The listing builds one solid part. Answer for the finished solid, in the listing's coordinates (mm). A direction names the side the tool comes from. Coordinates: 2 decimals unless noted, no trailing zeros. Loops run counter-clockwise (first coordinate to the right, second up) from the corner with the lowest first, then second, coordinate; pieces in that order, holes last. Notation, with made-up numbers: (-40, 38.5) -> (11, 38.5) arc R10 cw to (11, 52.5) -> close; hole circle Ø10 at (-39.75, 51.25). An arc over 180 degrees is marked (long way). Answer in a Markdown table with one row per item.
```python
from build123d import *

# Parameters (mm, degrees)
BOSS_EXTRUDE1_DEPTH      = 1.2
SKETCH2_R                = 1.5
CUT_EXTRUDE1_DEPTH       = 19.437461864
BOSS_EXTRUDE2_DEPTH      = 2.5
BOSS_EXTRUDE3_DEPTH      = 5.5
BOSS_EXTRUDE3_DEPTH_BACK = 4.7
SKETCH6_W                = 0.5
SKETCH6_H                = 0.5
SKETCH7_W                = 16
SKETCH7_H                = 26.8
BOSS_EXTRUDE4_DEPTH      = 1.8
SKETCH8_W                = 1.5
SKETCH8_H                = 0.75
SKETCH8_W_2              = 0.75
SKETCH8_H_2              = 1.5
BOSS_EXTRUDE5_DEPTH      = 0.8
SKETCH10_W               = 0.1
SKETCH10_H               = 8
BOSS_EXTRUDE6_DEPTH      = 0.1
SKETCH12_W               = 1
SKETCH12_H               = 22.2
BOSS_EXTRUDE7_DEPTH      = 0.06


with BuildPart() as part:
    # Sketch1 → Boss-Extrude1 (new body)
    with BuildSketch(Plane.XY):
        Polygon((10, -8.5), (10, 8.5), (12.5, 8.5), (12.5, 13.5), (-12.5, 13.5), (-12.5, -13.5), (12.5, -13.5), (12.5, -8.5), align=None)
    extrude(amount=BOSS_EXTRUDE1_DEPTH)

    # Sketch2 → Cut-Extrude1 (cut, through all)
    with BuildSketch(Plane.XY.offset(1.2)):
        with Locations((10.5, 11.5)):
            Circle(SKETCH2_R)
        with Locations(Location((10.5, -11.5, 0), (0, 0, 180))):
            Circle(SKETCH2_R)
        with Locations(Location((-10.5, 11.5, 0), (0, 0, 180))):
            Circle(SKETCH2_R)
        with Locations((-10.5, -11.5)):
            Circle(SKETCH2_R)
    extrude(amount=-CUT_EXTRUDE1_DEPTH, mode=Mode.SUBTRACT)

    # Sketch5 → Boss-Extrude2 (add)
    with BuildSketch(Plane(origin=(0, 0, 0), x_dir=(-1, 0, 0), z_dir=(0, 0, -1))):
        with BuildLine():
            Line((12.05, 6), (9.95, 6))
            ThreePointArc((9.95, 6), (9.808578644, 5.941421356), (9.75, 5.8))
            Line((9.75, 5.8), (9.75, 3.7))
            ThreePointArc((9.75, 3.7), (9.808578644, 3.558578644), (9.95, 3.5))
            ThreePointArc((9.95, 3.5), (9.808578644, 3.441421356), (9.75, 3.3))
            Line((9.75, 3.3), (9.75, 1.2))
            ThreePointArc((9.75, 1.2), (9.808578644, 1.058578644), (9.95, 1))
            ThreePointArc((9.95, 1), (9.808578644, 0.941421356), (9.75, 0.8))
            Line((9.75, 0.8), (9.75, -1.3))
            ThreePointArc((9.75, -1.3), (9.808578644, -1.441421356), (9.95, -1.5))
            ThreePointArc((9.95, -1.5), (9.808578644, -1.558578644), (9.75, -1.7))
            Line((9.75, -1.7), (9.75, -3.8))
            ThreePointArc((9.75, -3.8), (9.808578644, -3.941421356), (9.95, -4))
            Line((9.95, -4), (12.05, -4))
            ThreePointArc((12.05, -4), (12.191421356, -3.941421356), (12.25, -3.8))
            Line((12.25, -3.8), (12.25, -1.7))
            ThreePointArc((12.25, -1.7), (12.191421356, -1.558578644), (12.05, -1.5))
            ThreePointArc((12.05, -1.5), (12.191421356, -1.441421356), (12.25, -1.3))
            Line((12.25, -1.3), (12.25, 0.8))
            ThreePointArc((12.25, 0.8), (12.191421356, 0.941421356), (12.05, 1))
            ThreePointArc((12.05, 1), (12.191421356, 1.058578644), (12.25, 1.2))
            Line((12.25, 1.2), (12.25, 3.3))
            ThreePointArc((12.25, 3.3), (12.191421356, 3.441421356), (12.05, 3.5))
            ThreePointArc((12.05, 3.5), (12.191421356, 3.558578644), (12.25, 3.7))
            Line((12.25, 3.7), (12.25, 5.8))
            ThreePointArc((12.25, 5.8), (12.191421356, 5.941421356), (12.05, 6))
        make_face()
    extrude(amount=BOSS_EXTRUDE2_DEPTH)

    # Sketch6 → Boss-Extrude3 (add, two sides: drawn at the far end of the back side and taken through both)
    with BuildSketch(Plane(origin=(0, 0, -2.5), x_dir=(-1, 0, 0), z_dir=(0, 0, -1)).offset(-BOSS_EXTRUDE3_DEPTH_BACK)):
        with Locations((11, 4.75)):
            Rectangle(SKETCH6_W, SKETCH6_H)
        with Locations((11, 2.25)):
            Rectangle(SKETCH6_W, SKETCH6_H)
        with Locations((11, -0.25)):
            Rectangle(SKETCH6_W, SKETCH6_H)
        with Locations((11, -2.75)):
            Rectangle(SKETCH6_W, SKETCH6_H)
    extrude(amount=BOSS_EXTRUDE3_DEPTH + BOSS_EXTRUDE3_DEPTH_BACK)

    # Sketch7 → Boss-Extrude4 (add)
    with BuildSketch(Plane.XY.offset(1.2)):
        Rectangle(SKETCH7_W, SKETCH7_H)
    extrude(amount=BOSS_EXTRUDE4_DEPTH)

    # Sketch8 → Boss-Extrude5 (add)
    with BuildSketch(Plane(origin=(0, 0, 0), x_dir=(-1, 0, 0), z_dir=(0, 0, -1))):
        with Locations((0.75, 12.125)):
            Rectangle(SKETCH8_W, SKETCH8_H)
        with Locations((0.75, 9.402777778)):
            Rectangle(SKETCH8_W, SKETCH8_H)
        with Locations((0.75, 6.680555556)):
            Rectangle(SKETCH8_W, SKETCH8_H)
        with Locations((0.75, 3.958333333)):
            Rectangle(SKETCH8_W, SKETCH8_H)
        with Locations((0.75, 1.236111111)):
            Rectangle(SKETCH8_W, SKETCH8_H)
        with Locations((0.75, -1.486111111)):
            Rectangle(SKETCH8_W, SKETCH8_H)
        with Locations((0.75, -4.208333333)):
            Rectangle(SKETCH8_W, SKETCH8_H)
        with Locations((0.75, -6.930555556)):
            Rectangle(SKETCH8_W, SKETCH8_H)
        with Locations((0.75, -9.652777778)):
            Rectangle(SKETCH8_W, SKETCH8_H)
        with Locations((0.75, -12.375)):
            Rectangle(SKETCH8_W, SKETCH8_H)
        with Locations((-2.375, -9.75)):
            Rectangle(SKETCH8_W_2, SKETCH8_H_2)
        with Locations((-4.125, -9.75)):
            Rectangle(SKETCH8_W_2, SKETCH8_H_2)
        with Locations((-2.375, 9.75)):
            Rectangle(SKETCH8_W_2, SKETCH8_H_2)
        with Locations((-4.125, 9.75)):
            Rectangle(SKETCH8_W_2, SKETCH8_H_2)
    extrude(amount=BOSS_EXTRUDE5_DEPTH)

    # Sweep1: sweep along a path in Sketch9
    with BuildLine(Plane(origin=(0, 13.5, 0), x_dir=(1, 0, 0), z_dir=(0, 1, 0))) as sweep1_path:
        Line((8, -2.1), (10.5, -2.1))
        ThreePointArc((10.5, -2.1), (11.207106781, -1.807106781), (11.5, -1.1))
        Line((11.5, -1.1), (11.5, -0.95))
        ThreePointArc((11.5, -0.95), (11.207106781, -0.242893219), (10.5, 0.05))
        Line((10.5, 0.05), (9, 0.05))
    # Sketch10 → Sweep1 (sweep)
    with BuildSketch(Plane(origin=(8, 0, 0), x_dir=(0, 0, -1), z_dir=(1, 0, 0))):
        with Locations((-2.1, 0)):
            Rectangle(SKETCH10_W, SKETCH10_H)
    sweep(path=sweep1_path.line)

    # Sketch11 → Boss-Extrude6 (add)
    with BuildSketch(Plane(origin=(0, 0, 0), x_dir=(-1, 0, 0), z_dir=(0, 0, -1))):
        Polygon((-6.5, -11.1), (-6.5, 11.1), (-6.572413793, 11.1), (-10, 4), (-9, 4), (-9, -4), (-10, -4), (-6.572413793, -11.1), align=None)
    extrude(amount=BOSS_EXTRUDE6_DEPTH)

    # Sketch12 → Boss-Extrude7 (add)
    with BuildSketch(Plane(origin=(0, 0, 0), x_dir=(-1, 0, 0), z_dir=(0, 0, -1))):
        with Locations((-6, 0)):
            Rectangle(SKETCH12_W, SKETCH12_H)
    extrude(amount=BOSS_EXTRUDE7_DEPTH)


solid = part.part
```
Item 1: A cutting plane is placed at B-B, the plane y = -11.5. Determine the outline of the cut face in (x, z), plus the area to 3 significant figures.
Findings below:
| item | result |
|---|---|
| outline | (-12.5, 0) -> (-12, 0) -> (-12, 1.2) -> (-12.5, 1.2) -> close; (-9, 0) -> (9, 0) -> (9, 1.2) -> (8, 1.2) -> (8, 3) -> (-8, 3) -> (-8, 1.2) -> (-9, 1.2) -> close; (12, 0) -> (12.5, 0) -> (12.5, 1.2) -> (12, 1.2) -> close |
| area | 51.6 mm2 |
Item 2: Find the intervals of material crossed by probe 1 along Y at (x, z) = (10.5, 0.6); probe 2 along Y at (x, z) = (-10.5, 0.45); probe 3 along X at (y, z) = (5, -2), in increasing order.
Findings below:
| item | result |
|---|---|
| probe 1 | y = -13.5 to -13, -10 to -8.5, 8.5 to 10, 13 to 13.5 |
| probe 2 | y = -13.5 to -13, -10 to 10, 13 to 13.5 |
| probe 3 | x = -12.25 to -9.75 |
Item 3: A cutting plane is placed at D-D, the plane x = -7.5. Determine the outline of the cut face in (y, z).
Findings below:
| item | result |
|---|---|
| outline | (-13.5, 0) -> (13.5, 0) -> (13.5, 1.2) -> (13.4, 1.2) -> (13.4, 3) -> (-13.4, 3) -> (-13.4, 1.2) -> (-13.5, 1.2) -> close |
Item 4: Flat-ended cylindrical pins translate along their axes: pin 1 Ø1 at (y, z) = (2.5, -1) entering from -X; pin 2 Ø0.9 at (x, z) = (-0.5, -0.5) entering from +Y; pin 3 Ø0.9 at (y, z) = (-1, 2) entering from +X. Find the tip coordinate at first contact, or state that the pin passes through.
Findings below:
| item | result |
|---|---|
| pin 1 | stops at x = -12.25 |
| pin 2 | stops at y = 12.5 |
| pin 3 | stops at x = 11.45 |
Item 5: A tool of negligible diameter and unlimited length cuts with its end or side. For faces 4 (the face through (11, -8.5, 1)), 5 (the face through (0, 13.4, 2)), 6 (the face through (6, 0, -0.06)), 7 (the face through (-11, -4, -1)), 8 (the face through (-12.25, 2, -1)), from which of +Z, -Z, +X, -X, +Y, -Y can it reach the whole face along a straight path? Write none if from no direction.
Findings below:
| item | result |
|---|---|
| face 4 | +Z, -Z, +X |
| face 5 | +Z, +X, -X, +Y |
| face 6 | -Z, +Y, -Y |
| face 7 | -Z, -X, -Y |
| face 8 | -Z, -X, +Y, -Y |
Item 6: Determine the mould class of faces 1 (the face through (-12.25, 5, -1)), 2 (the face through (0, -13.4, 2)), 3 (the face through (-11.7, -12.4, 0.6)) for opening direction X: +X half, -X half, draft (parallel to the pull), parting line (faces both ways), or undercut.
Findings below:
| item | result |
|---|---|
| face 1 | -X half |
| face 2 | draft |
| face 3 | undercut |
Item 7: A cutting plane is placed at A-A, the plane z = -7. Determine the outline of the cut face in (x, y).
Findings below:
| item | result |
|---|---|
| outline | (-11.25, -3) -> (-10.75, -3) -> (-10.75, -2.5) -> (-11.25, -2.5) -> close; (-11.25, -0.5) -> (-10.75, -0.5) -> (-10.75, 0) -> (-11.25, 0) -> close; (-11.25, 2) -> (-10.75, 2) -> (-10.75, 2.5) -> (-11.25, 2.5) -> close; (-11.25, 4.5) -> (-10.75, 4.5) -> (-10.75, 5) -> (-11.25, 5) -> close |
Item 8: A cutting plane is placed at C-C, the plane x = 9.5. Determine the outline of the cut face in (y, z).
Findings below:
| item | result |
|---|---|
| outline | (-13.5, 0) -> (-12.62, 0) -> (-12.62, 1.2) -> (-13.5, 1.2) -> close; (-10.38, 0) -> (-5.04, 0) -> (-5.04, -0.1) -> (5.04, -0.1) -> (5.04, 0) -> (10.38, 0) -> (10.38, 1.2) -> (-10.38, 1.2) -> close; (-4, 2.05) -> (4, 2.05) -> (4, 2.15) -> (-4, 2.15) -> close; (12.62, 0) -> (13.5, 0) -> (13.5, 1.2) -> (12.62, 1.2) -> close |
